from build123d import *

# Parameters (mm, degrees)
SKETCH1_R           = 12.4
BOSS_EXTRUDE1_DEPTH = 20.9
SKETCH4_R           = 3.4
BOSS_EXTRUDE3_DEPTH = 2
SKETCH6_R           = 1.95
BOSS_EXTRUDE4_DEPTH = 11
CUT_EXTRUDE1_DEPTH  = 10
SKETCH8_R           = 12.1
BOSS_EXTRUDE5_DEPTH = 46.9
SKETCH9_R           = 1.5
CUT_EXTRUDE2_DEPTH  = 5
SKETCH10_W          = 13
SKETCH10_H          = 7.5
CUT_EXTRUDE3_DEPTH  = 4


with BuildPart() as part:
    # Sketch1 → Boss-Extrude1 (new body)
    with BuildSketch(Plane(origin=(0, 0, 0), x_dir=(1, 0, 0), z_dir=(0, 1, 0))):
        with Locations(Location((0, 0, 0), (0, 0, 270))):
            Circle(SKETCH1_R)
    extrude(amount=BOSS_EXTRUDE1_DEPTH)

    # Sketch4 → Boss-Extrude3 (add)
    with BuildSketch(Plane(origin=(0, 20.9, 0), x_dir=(1, 0, 0), z_dir=(0, 1, 0))):
        with Locations(Location((0, 0, 0), (0, 0, 270))):
            Circle(SKETCH4_R)
    extrude(amount=BOSS_EXTRUDE3_DEPTH)

    # Sketch6 → Boss-Extrude4 (add)
    with BuildSketch(Plane(origin=(0, 22.9, 0), x_dir=(1, 0, 0), z_dir=(0, 1, 0))):
        with Locations(Location((0, 0, 0), (0, 0, 270))):
            Circle(SKETCH6_R)
    extrude(amount=BOSS_EXTRUDE4_DEPTH)

    # Sketch7 → Cut-Extrude1 (cut)
    with BuildSketch(Plane(origin=(0, 33.9, 0), x_dir=(1, 0, 0), z_dir=(0, 1, 0))):
        Polygon((0, 1.45), (-1.840503263, 1.45), (-1.840503263, 3.329277937), (1.844863843, 3.329277937), (1.844863843, 1.45), align=None)
    extrude(amount=-CUT_EXTRUDE1_DEPTH, mode=Mode.SUBTRACT)

    # Sketch8 → Boss-Extrude5 (add)
    with BuildSketch(Plane.XZ):
        with Locations(Location((0, 0, 0), (0, 0, 270))):
            Circle(SKETCH8_R)
    extrude(amount=BOSS_EXTRUDE5_DEPTH)

    # Sketch9 → Cut-Extrude2 (cut)
    with BuildSketch(Plane(origin=(0, 20.9, 0), x_dir=(1, 0, 0), z_dir=(0, 1, 0))):
        with Locations(Location((-8.1, 0, 0), (0, 0, 270))):
            Circle(SKETCH9_R)
        with Locations(Location((8.1, 0, 0), (0, 0, 90))):
            Circle(SKETCH9_R)
    extrude(amount=-CUT_EXTRUDE2_DEPTH, mode=Mode.SUBTRACT)

    # Sketch10 → Cut-Extrude3 (cut)
    with BuildSketch(Plane.XY.offset(13)):
        with Locations((0, -34.15)):
            Rectangle(SKETCH10_W, SKETCH10_H)
    extrude(amount=-CUT_EXTRUDE3_DEPTH, mode=Mode.SUBTRACT)


solid = part.part
The listing builds one solid part. Answer for the finished solid, in the listing's coordinates (mm). A direction names the side the tool comes from. Coordinates: 2 decimals unless noted, no trailing zeros. Loops run counter-clockwise (first coordinate to the right, second up) from the corner with the lowest first, then second, coordinate; pieces in that order, holes last.
1) Determine the mould class of faces 6 (the face through (-8, 15.9, 0)), 7 (the face through (0, -46.9, 0)), 8 (the face through (8, 15.9, 0)), 9 (the face through (-3.32, 21.89, -0.74)) for opening direction X: pulls with the +X half, pulls with the -X half, needs draft (parallel to the pull), parting line crosses it, or undercut.
2) Flat-ended cylindrical pins translate along their axes: pin 1 Ø1.5 at (x, z) = (-8, 0) entering from +Y; pin 2 Ø5 at (y, z) = (-5, 1.5) entering from -X; pin 3 Ø5 at (y, z) = (2.5, -7) entering from -X. Find the tip coordinate at first contact, or state that the pin passes through.
3) Find section A-A on x = 0. Write down the section's boundary in (y, z), then the cut area to 3 significant figures.
4) A tool of negligible diameter and unlimited length cuts with its end or side. For faces 1 (the face through (0, -34, 9)), 2 (the face through (6.613, 18.435, 0.195)), 3 (the face through (0, 29, -1.45)), 4 (the face through (0, 33.9, 0)), 5 (the face through (3.635, -23.122, -11.541)), from which of +Z, -Z, +X, -X, +Y, -Y can it reach the whole face along a straight path? Write none if from no direction.
5) Find section B-B on z = 0. Write down the section's boundary in (x, y).
6) Find section D-D on y = -20. Write down the section's boundary in (x, z), then the cut area to 3 significant figures.
7) Find section C-C on y = 13. Write down the section's boundary in (x, z), then the cut area to 3 significant figures.
8) Find the intervals of material crossed by L1, parallel to Y at x = -4, z = -1.75; L2, parallel to Z at x = 8.1, y = 18.65; L3, parallel to Y at x = -3, z = -0.75, in increasing order.
Values:
1. face 6: undercut
1. face 7: needs draft
1. face 8: undercut
1. face 9: parting line crosses it
2. pin 1: stops at y = 15.9
2. pin 2: stops at x = -12.1
2. pin 3: stops at x = -11.55
3. outline: (-46.9, -12.1) - (0, -12.1) - (0, -12.4) - (20.9, -12.4) - (20.9, -3.4) - (22.9, -3.4) - (22.9, -1.95) - (23.9, -1.95) - (23.9, -1.45) - (33.9, -1.45) - (33.9, 1.95) - (22.9, 1.95) - (22.9, 3.4) - (20.9, 3.4) - (20.9, 12.4) - (0, 12.4) - (0, 12.1) - (-30.4, 12.1) - (-30.4, 9) - (-37.9, 9) - (-37.9, 12.1) - (-46.9, 12.1) - close
3. area: 1,680 mm2
4. face 1: +Z
4. face 2: +Y
4. face 3: -Z, +X, -X, +Y
4. face 4: +Z, -Z, +X, -X, +Y
4. face 5: -Y
5. outline: (-12.4, 0) - (-12.1, 0) - (-12.1, -46.9) - (12.1, -46.9) - (12.1, 0) - (12.4, 0) - (12.4, 20.9) - (9.6, 20.9) - (9.6, 15.9) - (6.6, 15.9) - (6.6, 20.9) - (3.4, 20.9) - (3.4, 22.9) - (1.95, 22.9) - (1.95, 33.9) - (-1.95, 33.9) - (-1.95, 22.9) - (-3.4, 22.9) - (-3.4, 20.9) - (-6.6, 20.9) - (-6.6, 15.9) - (-9.6, 15.9) - (-9.6, 20.9) - (-12.4, 20.9) - close
6. outline: circle Ø24.2 at (0, 0)
6. area: 460 mm2
7. outline: circle Ø24.8 at (0, 0)
7. area: 483 mm2
8. L1: y = -46.9 to 20.9
8. L2: z = -9.39 to -1.5, 1.5 to 9.39
8. L3: y = -46.9 to 22.9
